from build123d import *

# Parameters (mm, degrees)
SKETCH4_R           = 2
BOSS_EXTRUDE1_DEPTH = 0.5
CUT_EXTRUDE1_REACH  = 68.966
SKETCH6_R           = 8.04


with BuildPart() as part:
    # Sweep1: sweep along a path in Sketch2
    with BuildLine(Plane.XY) as sweep1_path:
        Line((0, 0), (0, -83))
        ThreePointArc((0, -83), (-0.841224391, -89.596719602), (-3.311053985, -95.771208226))
        Line((-3.311053985, -95.771208226), (-14, -115))
    # Sketch4 → Sweep1 (sweep)
    with BuildSketch(Plane(origin=(0, 0, 0), x_dir=(1, 0, 0), z_dir=(0, 1, 0))):
        Circle(SKETCH4_R)
    sweep(path=sweep1_path.line)

    # Sketch5 → Boss-Extrude1 (add, symmetric)
    with BuildSketch(Plane(origin=(0, -60, 0), x_dir=(1, 0, 0), z_dir=(0, 1, 0))):
        with BuildLine():
            Line((-18.84, -10.16), (-12.115048494, -10.16))
            Line((-12.115048494, -10.16), (1.836495151, -4.650514548))
            ThreePointArc((1.836495151, -4.650514548), (4.650514548, 1.836495151), (-1.836495151, 4.650514548))
            Line((-1.836495151, 4.650514548), (-8.855227327, 1.878806714))
            ThreePointArc((-8.855227327, 1.878806714), (-26.660302942, 6.486020497), (-18.84, -10.16))
        make_face()
    extrude(amount=BOSS_EXTRUDE1_DEPTH, both=True)

    # Sketch6 → Cut-Extrude1 (cut, up to next)
    with BuildSketch(Plane(origin=(0, -59.5, 0), x_dir=(1, 0, 0), z_dir=(0, 1, 0)), mode=Mode.PRIVATE) as cut_extrude1_sk1:
        with Locations(Location((-18.84, 0, 0), (0, 0, 270))):
            Circle(SKETCH6_R)
    cut_extrude1_tool1 = extrude(cut_extrude1_sk1.sketch, amount=-CUT_EXTRUDE1_REACH, mode=Mode.PRIVATE) & part.part
    add(cut_extrude1_tool1.solids().sort_by_distance((-18.84, -59.5, 0))[0], mode=Mode.SUBTRACT)


solid = part.part
CAD build for the part. Positions are in the model's coordinates, mm. A direction names the side the tool comes from. Give positions to 0.01 mm unless a question says otherwise; leave off trailing zeros. Write each loop counter-clockwise with the first axis right and the second up, starting at its lowest first coordinate (ties: lowest second). Pieces come first, ordered by that corner, then holes. Notation, with made-up numbers: (-21.75, -35) - (17.25, -35) arc R28 ccw to (17.25, -2) - close; hole circle Ø1 at (44.5, -3.5). An arc over 180 degrees is marked (long way). Answer as CSV lines item,"result".
Q1. Band-saw the part on D-D (z = -6). Give the cut face in (x, y), and give its area (3 significant figures).
Result set:
outline,"(-27.04, -60.5) - (-24.19, -60.5) - (-24.19, -59.5) - (-27.04, -59.5) - close; (-13.49, -60.5) - (-10.64, -60.5) - (-10.64, -59.5) - (-13.49, -59.5) - close"
area,"5.69 mm²"
Q2. Band-saw the part on A-A (z = 0). Give the cut face in (x, y).
Result set:
outline,"(-29, -60.5) - (-26.88, -60.5) - (-26.88, -59.5) - (-29, -59.5) - close; (-15.75, -114.03) - (-12.25, -115.97) - (-1.56, -96.74) arc R28.29 ccw to (2, -83) - (2, -60.5) - (5, -60.5) - (5, -59.5) - (2, -59.5) - (2, 0) - (-2, 0) - (-2, -59.5) - (-10.8, -59.5) - (-10.8, -60.5) - (-2, -60.5) - (-2, -83) arc R24.29 cw to (-5.06, -94.8) - close"
Q3. Drill centre lines: line 1 (X direction, y = -60.2, z = 0); line 2 (Z direction, x = -18, y = -60); line 3 (Y direction, x = -7, z = 6.25). Where is each one in solid material? Low to high. Write a range as from..to.
Result set:
line 1,"-29..-26.88, -10.8..5"
line 2,"-10.13..-8, 8..10.16"
line 3,"-60.5..-59.5"
Q4. Band-saw the part on B-B (z = 6.25). Give the cut face in (x, y).
Result set:
outline,"(-26.85, -60.5) - (-23.9, -60.5) - (-23.9, -59.5) - (-26.85, -59.5) - close; (-13.78, -60.5) - (-2.21, -60.5) - (-2.21, -59.5) - (-13.78, -59.5) - close"
Q5. 3-axis set-ups, long thin cutter, end or side, ignore diameter. For faces 5 (the face through (0, -30, -2)), 6 (the face through (-5.237, -59.993, 7.444)): which of +Z, -Z, +X, -X, +Y, -Y reach the whole face in a straight line?
Result set:
face 5,"+Y"
face 6,"+Z, +X, +Y, -Y"
Q6. Pull direction Y, two halves, no side cores. Call faces 1 (the face through (-8, -59.5, 2)), 2 (the face through (0, -72, -2)), 3 (the face through (-26.45, -59.99, -6.73)), 4 (the face through (-14, -115, 0)): released by +Y, released by -Y, zero draft, split by the parting line, or undercut.
Result set:
face 1,"released by +Y"
face 2,"undercut"
face 3,"zero draft"
face 4,"released by -Y"
Q7. Flat gauge pins, fed straight in: pin 1 Ø6 at (x, z) = (-8.5, -1.5) entering from -Y; pin 2 Ø10 at (x, z) = (-7, 4) entering from +Y; pin 3 Ø6 at (y, z) = (-89, -3) entering from -X; pin 4 Ø5 at (y, z) = (-52, 6) entering from +X. Where does each tip first touch, or does it go through?
Result set:
pin 1,"y = -114.18"
pin 2,"y = -59.5"
pin 3,"x = -3.2"
pin 4,"through"
Q8. Band-saw the part on C-C (y = -71.5). Give the cut face in (x, z).
Result set:
outline,"circle Ø4 at (0, 0)"
